Source: CAD feature listing. Evaluate the final solid. Frame: model axes, mm. A direction names the side the tool comes from. Give positions to 0.01 mm unless a question says otherwise; leave off trailing zeros. Write each loop counter-clockwise with the first axis right and the second up, starting at its lowest first coordinate (ties: lowest second). Pieces come first, ordered by that corner, then holes. Notation, with made-up numbers: (46, 43) -> (64, 43) arc R12 ccw to (64, 57) -> close; hole circle Ø9 at (17.25, 62.25). An arc over 180 degrees is marked (long way). Answer as a JSON object with one key per item and string values. Group by question number.
Item 1: Ray query, probe 1 along X at (y, z) = (-43, 11.6); probe 2 along Z at (x, y) = (-20.5, -44.5). Return the intervals inside material, ascending. Write a range as from..to.
Item 2: Pull-direction query (Z, two-part tool) for faces 1 (the face through (-9.138, -2.878, 132.307)), 2 (the face through (16.8, 46.16, 87.54)), 3 (the face through (-35.334, -3.048, 74.391)), 4 (the face through (-48.289, -48.196, 11.521)); classes: pulls with the +Z half, pulls with the -Z half, needs draft (parallel to the pull), parting line crosses it, or undercut.
Item 3: Section query B-B on z = 106. Return the cut outline in (x, y).
Item 4: Access query for faces 5 (the face through (24.56, -42.54, 87.54)), 6 (the face through (20.7, 29.56, 75.35)). Directions: +Z, -Z, +X, -X, +Y, -Y. A direction counts if a zero-diameter tool reaches every point of the face in a straight line with its end or side. Return the directions, or none.
Item 5: First-contact query: pin 1 Ø4.5 at (x, y) = (23, 46.5) entering from +Z; pin 2 Ø2.5 at (x, y) = (2.5, 37.5) entering from +Z; pin 3 Ø1 at (x, y) = (-23.5, -14) entering from +Z. Flat tips, straight axial feed; report the tip coordinate or a pass-through.
Item 6: Section query A-A on y = 14. Give the number of separate pieces and of enclosed holes in the cut face, plus the area to 3 significant figures.
from build123d import *

# Parameters (mm, degrees)
SKETCH006_R           = 40
SKETCH006_R_2         = 38
PAD002_DEPTH          = 50
SKETCH007_R           = 42
SKETCH007_R_2         = 40
PAD003_DEPTH          = 40
SKETCH019_W           = 100
SKETCH019_H           = 100
SKETCH019_R           = 40
PAD010_DEPTH          = 3
FILLET001_R           = 6
SKETCH020_R           = 3
POCKET004_DEPTH       = 3
CHAMFER_SIZE          = 1.9
CHAMFER002_SIZE       = 1.9
REVOLUTION_ANGLE      = 10
POLARPATTERN_COUNT    = 8
SKETCH022_W           = 20
SKETCH022_H           = 5
REVOLUTION004_ANGLE   = 10
POLARPATTERN006_COUNT = 6
SKETCH024_R           = 60
SKETCH024_R_2         = 58
PAD011_DEPTH          = 40
SKETCH030_R           = 40.5
POCKET006_DEPTH       = 30


with BuildPart() as part:
    # Sketch006 → Pad002 (new body)
    with BuildSketch(Plane.XY):
        Circle(SKETCH006_R)
        Circle(SKETCH006_R_2, mode=Mode.SUBTRACT)
    extrude(amount=PAD002_DEPTH)

    # Sketch007 (on Face3 of Pad002) → Pad003 (join)
    with BuildSketch(Plane(origin=(0, 0, 10), x_dir=(1, 0, 0), z_dir=(0, 0, -1))):
        Circle(SKETCH007_R)
        Circle(SKETCH007_R_2, mode=Mode.SUBTRACT)
    extrude(amount=PAD003_DEPTH)

    # Sketch019 (on Face6 of Pad003) → Pad010 (join)
    with BuildSketch(Plane(origin=(0, 0, -30), x_dir=(1, 0, 0), z_dir=(0, 0, -1))):
        Rectangle(SKETCH019_W, SKETCH019_H)
        Circle(SKETCH019_R, mode=Mode.SUBTRACT)
    extrude(amount=-PAD010_DEPTH)

    # Fillet001
    fillet001_edges = [part.edges().sort_by_distance(p)[0] for p in [
        (-50, 50, -28.5),
        (-50, -50, -28.5),
        (50, -50, -28.5),
        (50, 50, -28.5),
    ]]
    fillet(fillet001_edges, radius=FILLET001_R)

    # Sketch020 (on Face11 of Fillet001) → Pocket004 (cut)
    with BuildSketch(Plane(origin=(0, 0, -30), x_dir=(1, 0, 0), z_dir=(0, 0, -1))):
        with Locations((-43, 43)):
            Circle(SKETCH020_R)
        with Locations((43, 43)):
            Circle(SKETCH020_R)
        with Locations((43, -43)):
            Circle(SKETCH020_R)
        with Locations((-43, -43)):
            Circle(SKETCH020_R)
    extrude(amount=-POCKET004_DEPTH, mode=Mode.SUBTRACT)

    # Chamfer
    chamfer_edges = [part.edges().sort_by_distance(p)[0] for p in [
        (-38, 0, 0),
    ]]
    chamfer(chamfer_edges, length=CHAMFER_SIZE)

    # Chamfer002
    chamfer002_edges = [part.edges().sort_by_distance(p)[0] for p in [
        (-42, 0, 10),
    ]]
    chamfer(chamfer002_edges, length=CHAMFER002_SIZE)

    # Sketch021 → Revolution (revolve)
    with BuildSketch(Plane.YZ):
        Polygon((-38, 38.660254), (-38, 30), (-33, 38.660254), align=None)
    revolution = revolve(axis=Axis((0, 0, 0), (0, 0, 1)), revolution_arc=REVOLUTION_ANGLE)

    # PolarPattern: Revolution ×8 about axis
    polarpattern_axis = Axis((0, 0, 0), (0, 0, 1))
    for i in range(1, POLARPATTERN_COUNT):
        add(revolution.rotate(polarpattern_axis, i * 360 / POLARPATTERN_COUNT))

    # Sketch022 → Revolution004 (revolve)
    with BuildSketch(Plane.XZ):
        with Locations((-50, 47.5)):
            Rectangle(SKETCH022_W, SKETCH022_H)
        with Locations((-50, 12.5)):
            Rectangle(SKETCH022_W, SKETCH022_H)
    revolution004 = revolve(axis=Axis((0, 0, 0), (0, 0, 1)), revolution_arc=REVOLUTION004_ANGLE)

    # PolarPattern006: Revolution004 ×6 about axis
    polarpattern006_axis = Axis((0, 0, 0), (0, 0, 1))
    for i in range(1, POLARPATTERN006_COUNT):
        add(revolution004.rotate(polarpattern006_axis, i * 360 / POLARPATTERN006_COUNT))

    # Sketch023 → Revolution005 (revolve)
    with BuildSketch(Plane.XZ):
        Polygon((-60, 50), (0, 100.345978), (0, 98.667779), (-58, 50), align=None)
    revolve(axis=Axis((0, 0, 0), (0, 0, 1)))

    # Sketch024 (on Face68 of Revolution005) → Pad011 (join)
    with BuildSketch(Plane(origin=(0, 0, 50), x_dir=(1, 0, 0), z_dir=(0, 0, -1))):
        Circle(SKETCH024_R)
        Circle(SKETCH024_R_2, mode=Mode.SUBTRACT)
    extrude(amount=PAD011_DEPTH)

    # Sketch030 (on Face135 of Pad011) → Pocket006 (cut)
    with BuildSketch(Plane(origin=(0, 0, -30), x_dir=(1, 0, 0), z_dir=(0, 0, -1))):
        Circle(SKETCH030_R)
    extrude(amount=-POCKET006_DEPTH, mode=Mode.SUBTRACT)


with BuildPart() as part_1:
    # Body001 placement: moved
    add(part.part.moved(Location((0, 0, 40))))


solid = part_1.part
Worked answers:
{
 "1": {"probe 1": "-50..-46, -40..40, 46..50", "probe 2": "10..13, 50..55, 85..90, 97.56..99.23"},
 "2": {"face 1": "pulls with the +Z half", "face 2": "undercut", "face 3": "pulls with the -Z half", "face 4": "needs draft"},
 "3": {"outline": "circle Ø81.86 at (0, 0); hole circle Ø77.86 at (0, 0)"},
 "4": {"face 5": "none", "face 6": "-Z"},
 "5": {"pin 1": "z = 98.7", "pin 2": "z = 109.86", "pin 3": "z = 117.81"},
 "6": {"separate pieces": "3", "enclosed holes": "0", "area": "764 mm^2"}
}
